Autodesk Inventor part; units mm, degrees
ref_plane "Work Plane1" through (-46.8123, -99.7095, 22.225) normal (0, 0, -1) x (0, 1, 0)
ref_plane "YZ Plane" through (0, 0, 0) normal (1, 0, 0) x (0, 1, 0)
ref_plane "XZ Plane" through (0, 0, 0) normal (0, 1, 0) x (-1, 0, 0)
sketch "Sketch1" plane through (0, 0, 0) normal (0, 0, 1) x (1, 0, 0)
  arc A0 (-18.2373, -76.3503) -> (26.9537, -71.5105) centre (0, -33.2365) ccw
  line L0 (26.9537, -71.5105) -> (46.8123, -71.5105)
  line L1 (46.8123, -71.5105) -> (46.8123, -74.3095)
  arc A1 (23.0377, -99.6575) -> (46.8123, -74.3095) centre (21.4123, -74.3095) ccw
  line L2 (23.0377, -99.6575) -> (23.0377, -92.0895)
  line L3 (23.0377, -92.0895) -> (-18.2373, -92.0895)
  line L4 (-18.2373, -76.3503) -> (-18.2373, -92.0895)
  arc A2 (21.4123, -99.7095) -> (46.8123, -74.3095) centre (21.4123, -74.3095) ccw
  line L5 (46.8123, -74.3095) -> (46.8123, -71.5105)
  line L6 (46.8123, -71.5105) -> (26.9537, -71.5105)
  arc A3 (-26.9537, -71.5105) -> (26.9537, -71.5105) centre (0, -33.2365) ccw
  line L7 (-26.9537, -71.5105) -> (-46.8123, -71.5105)
  line L8 (-46.8123, -71.5105) -> (-46.8123, -74.3095)
  arc A4 (-46.8123, -74.3095) -> (-21.4123, -99.7095) centre (-21.4123, -74.3095) ccw
  line L9 (-21.4123, -99.7095) -> (21.4123, -99.7095)
  line L10 (-18.2373, -92.0895) -> (-18.2373, -99.7095)
  line L11 (-18.2373, -92.0895) -> (23.0377, -92.0895)
  line L12 (23.0377, -92.0895) -> (23.0377, -99.6575)
  point P0 (0, 0)
ref_plane "Work Plane1" through (-46.8123, -99.7095, 22.225) normal (0, 0, -1) x (0, 1, 0)
extrude "Extrusion1" add sketch "Sketch1" along normal up to surface (22.225 mm away) contours L3 L2 A2 L9 L10
sketch "Sketch2" plane through (-18.2373, -92.0895, 22.225) normal (0, 1, 0) x (1, 0, 0)
  circle A0 centre (39.0525, 2.4765) radius 1.27
  circle A1 centre (39.0525, 20.2565) radius 1.27
  circle A2 centre (10.4775, 20.2565) radius 1.27
  circle A3 centre (10.4775, 2.4765) radius 1.27
  circle A4 centre (39.0525, 2.4765) radius 1.143
  circle A5 centre (39.0525, 20.2565) radius 1.143
  circle A6 centre (10.4775, 2.4765) radius 1.143
  circle A7 centre (10.4775, 20.2565) radius 1.143
  point P0 (18.2373, 22.225)
  dimension "d4" = 0.127
  dimension "d5" = 0.127
  dimension "d6" = 0.127
  dimension "d7" = 0.127
extrude "Extrusion2" add sketch "Sketch2" along normal blind 6.096 contours A4 | A5 | A6 | A7
ref_plane "Work Plane2" through (-15.0623, -99.7095, 0) normal (-1, 0, 0) x (0, 0, 1)
sketch "Sketch3" plane through (-15.0623, -99.7095, 0) normal (-1, 0, 0) x (0, 0, 1)
  arc A0 (8.8042, -0.8832) -> (13.0521, -0.8802) centre (10.922, 7.62) ccw
  circle A1 centre (10.922, 7.62) radius 3.175
  line L0 (13.744, 9.3345) -> (17.399, 9.3345)
  line L1 (17.399, 9.3345) -> (17.399, 7.62)
  line L2 (17.399, 9.3345) -> (17.399, 5.9055)
  line L3 (17.399, 5.9055) -> (13.744, 5.9055)
  arc A2 (13.744, 9.3345) -> (13.744, 5.9055) centre (10.922, 7.62) ccw
  arc A3 (19.7485, 7.62) -> (1.9685, 7.62) centre (10.8585, 7.62) ccw
  arc A4 (1.9685, 7.62) -> (19.7485, 7.62) centre (10.8585, 7.62) ccw
  line L4 (19.7485, 7.62) -> (17.399, 7.62)
  line L5 (18.6055, 7.62) -> (20.8915, 7.62)
  line L6 (0, 7.62) -> (22.225, 7.62)
  line L7 (7.62, 7.62) -> (1.9685, 7.62)
  point P0 (0, 99.7095)
extrude "Extrusion3" cut sketch "Sketch3" against normal blind 5.08
pattern_linear "Rectangular Pattern1" count 4 spacing 9.525 along (1, 0, 0) of "Extrusion3"
sketch "Sketch4" plane through (-18.2373, -99.7095, 0) normal (-1, 0, 0) x (0, 0, 1)
  line L0 (17.399, 9.3345) -> (17.399, 5.9055)
  line L1 (17.399, 5.9055) -> (13.744, 5.9055)
  arc A0 (13.744, 9.3345) -> (13.744, 5.9055) centre (10.922, 7.62) ccw
  line L2 (1.9685, 7.62) -> (19.7485, 7.62)
  line L3 (17.399, 7.62) -> (7.62, 7.62)
  point P0 (0, 99.7095)
extrude "Extrusion4" cut sketch "Sketch4" against normal through all
properties part number "lock housing front"
Read the model definition and answer for the solid it produces. Units are mm, in the model's axes. A direction names the side the tool comes from. Give positions to 0.01 mm unless a question says otherwise; leave off trailing zeros. Loops run counter-clockwise (first coordinate to the right, second up) from the corner with the lowest first, then second, coordinate; pieces in that order, holes last.
Item 1: The part is cut by section A-A (x = -4). Write down the section's boundary in (y, z) (1 decimal).
Item 2: Each of these flat-tipped pins is pushed along its axis until it touches: pin 1 Ø4 at (x, z) = (11.5, 12) entering from +Y; pin 2 Ø0.5 at (x, y) = (2, -93) entering from -Z; pin 3 Ø5 at (y, z) = (-89.5, 19) entering from -X; pin 4 Ø6 at (x, z) = (0.5, 5) entering from +Y. Where does it stop, or does it pass through?
Item 3: The part is cut by section D-D (y = -98.5). Write down the section's boundary in (x, z) (3 decimals), and give its area (3 significant figures).
Item 4: The part is cut by section C-C (x = 1). Write down the section's boundary in (y, z) (1 decimal).
Item 5: Find the intervals of material crossed by line 1 along X through (y, z) = (-94.75, 19); line 2 along X through (y, z) = (-91.5, 2); line 3 along Z through (x, y) = (0, -93.5) (3 decimals), in increasing order.
Item 6: The part is cut by section B-B (z = 15). Write down the section's boundary in (x, y), and give its area (3 significant figures).
Item 7: For faces 5 (the flat face through (1, -99.71, 11)), 6 (the flat face through (11, -93.804, 16)), 7 (the flat face through (-15.062, -96, 11)), determine the directions among +Z, -Z, +X, -X, +Y, -Y from which every point of the face is accessible in a straight line to the end or side of a thin tool.
Item 8: The mould has two halves that part along X. Classify faces 1 (the flat face through (9.068, -96, 11)), 2 (the flat face through (-17, -93.804, 16)), 3 (the flat face through (23.038, -96, 11)), 4 (the flat face through (18.593, -96, 11)): released by +X, released by -X, zero draft, split by the parting line, or undercut.
Taken from the geometry:
1. outline: (-99.7, 0) - (-92.1, 0) - (-92.1, 2) arc R8.9 cw to (-99.7, 6.3) - close; (-99.7, 15.4) arc R8.9 cw to (-92.1, 19.7) - (-92.1, 22.2) - (-99.7, 22.2) - close
2. pin 1: stops at y = -93.8
2. pin 2: stops at z = 0
2. pin 3: stops at x = -8.9
2. pin 4: stops at y = -92.09
3. outline: (-18.237, 0) - (23.038, 0) - (23.038, 22.225) - (-18.237, 22.225) - close; hole (-15.062, 4.699) - (-9.982, 4.699) - (-9.982, 17.018) - (-15.062, 17.018) - close; hole (-5.537, 4.699) - (-0.457, 4.699) - (-0.457, 17.018) - (-5.537, 17.018) - close; hole (3.988, 4.699) - (9.068, 4.699) - (9.068, 17.018) - (3.988, 17.018) - close; hole (13.513, 4.699) - (18.593, 4.699) - (18.593, 17.018) - (13.513, 17.018) - close
3. area: 667 mm2
4. outline: (-99.7, 0) - (-92.1, 0) - (-92.1, 7.6) arc R3.3 cw to (-93.8, 13.7) - (-93.8, 17.4) - (-92.1, 17.4) - (-92.1, 22.2) - (-99.7, 22.2) - close
5. line 1: x = -18.24 to -15.06, -9.98 to -5.54, -0.46 to 3.99, 9.07 to 13.51, 18.59 to 23.04
5. line 2: x = -8.9 to -6.62, 19.67 to 21.96
5. line 3: z = 0 to 7.936, 17.399 to 22.225
6. outline: (-18.24, -99.71) - (-15.06, -99.71) - (-15.06, -93.8) - (-18.24, -93.8) - close; (-9.98, -99.71) - (-5.54, -99.71) - (-5.54, -93.8) - (-9.98, -93.8) - close; (-0.46, -99.71) - (3.99, -99.71) - (3.99, -93.8) - (-0.46, -93.8) - close; (9.07, -99.71) - (13.51, -99.71) - (13.51, -93.8) - (9.07, -93.8) - close; (18.59, -99.71) - (21.41, -99.71) arc R25.4 ccw to (23.04, -99.66) - (23.04, -93.8) - (18.59, -93.8) - close
6. area: 124 mm2
7. face 5: +Z, -Z, +X, -X, -Y
7. face 6: +X, -X, +Y
7. face 7: +Y
8. face 1: undercut
8. face 2: zero draft
8. face 3: released by +X
8. face 4: undercut
